Read the model definition and answer for the solid it produces. Units are mm, in the model's axes. A direction names the side the tool comes from. Coordinates: 2 decimals unless noted, no trailing zeros. Write each loop counter-clockwise with the first axis right and the second up, starting at its lowest first coordinate (ties: lowest second). Pieces come first, ordered by that corner, then holes. Notation, with made-up numbers: (19, 29) - (35, 29) arc R18 cw to (35, 34) - close; hole circle Ø2 at (56, 5.5). An arc over 180 degrees is marked (long way). Return JSON: item names as keys, results as strings.
```python
from build123d import *

# Parameters (mm, degrees)
SKETCH_1_W          = 151
SKETCH_1_H          = 95
EXTRUDE_1_DEPTH     = 1.6
SKETCH_2_W          = 41
SKETCH_2_H          = 4.6
EXTRUDE_2_DEPTH     = 151
SKETCH_3_R          = 1.5
CUT_EXTRUDE_1_DEPTH = 179.506134348


with BuildPart() as part:
    # 草图1 → 凸台-拉伸1 (new body)
    with BuildSketch(Plane(origin=(0, 0, 0), x_dir=(1, 0, 0), z_dir=(0, 1, 0))):
        with Locations((75.5, -47.5)):
            Rectangle(SKETCH_1_W, SKETCH_1_H)
    extrude(amount=EXTRUDE_1_DEPTH)

    # 草图2 → 凸台-拉伸2 (add)
    with BuildSketch(Plane.ZY):
        with Locations((47.5, -2.3)):
            Rectangle(SKETCH_2_W, SKETCH_2_H)
    extrude(amount=-EXTRUDE_2_DEPTH)

    # 草图3 → 切除-拉伸1 (cut, through all)
    with BuildSketch(Plane(origin=(0, 1.6, 0), x_dir=(1, 0, 0), z_dir=(0, 1, 0))):
        with Locations(Location((5.5, -5, 0), (0, 0, 270))):
            Circle(SKETCH_3_R)
        with Locations(Location((5.5, -90, 0), (0, 0, 270))):
            Circle(SKETCH_3_R)
        with Locations(Location((145.5, -90, 0), (0, 0, 270))):
            Circle(SKETCH_3_R)
        with Locations(Location((145.5, -5, 0), (0, 0, 270))):
            Circle(SKETCH_3_R)
    extrude(amount=-CUT_EXTRUDE_1_DEPTH, mode=Mode.SUBTRACT)


solid = part.part
```
(1) A cutting plane is placed at D-D (y = -1.5). Determine the outline of the cut face in (x, z).
Answer:
{"outline": "(0, 27) - (151, 27) - (151, 68) - (0, 68) - close"}
(2) Flat-ended cylindrical pins translate along their axes: P1, Ø1.4, axis at x = 44.5, y = -3.5, coming from the +Z side; P2, Ø2.5, axis at x = 5.5, z = 5, coming from the -Y side; P3, Ø1, axis at x = 98, y = -3, coming from the -Z side; P4, Ø4, axis at x = 145.5, z = 90, coming from the -Y side. Find the tip coordinate at first contact, or state that the pin passes through.
Answer:
{"P1": "z = 68", "P2": "through", "P3": "z = 27", "P4": "y = 0"}
(3) Straight lines are drawn through the part: line 1 (Z direction, x = 145.5, y = 0.95); line 2 (X direction, y = 1.05, z = 5); line 3 (Z direction, x = 25, y = -3.75). For each, find the intervals that lie inside material, in ascending order. Write a range as from..to.
Answer:
{"line 1": "0..3.5, 6.5..88.5, 91.5..95", "line 2": "0..4, 7..144, 147..151", "line 3": "27..68"}
(4) A cutting plane is placed at C-C (z = 16). Determine the outline of the cut face in (x, y), and give its area (3 significant figures).
Answer:
{"outline": "(0, 0) - (151, 0) - (151, 1.6) - (0, 1.6) - close", "area": "242 mm²"}
(5) A cutting plane is placed at B-B (z = 90). Determine the outline of the cut face in (x, y).
Answer:
{"outline": "(0, 0) - (4, 0) - (4, 1.6) - (0, 1.6) - close; (7, 0) - (144, 0) - (144, 1.6) - (7, 1.6) - close; (147, 0) - (151, 0) - (151, 1.6) - (147, 1.6) - close"}
(6) Determine the mould class of faces 1 (the face through (151, -1, 48)), 2 (the face through (146.765, 0.811, 90.806)), 3 (the face through (74, 0, 13)) for opening direction X: +X half, -X half, draft (parallel to the pull), parting line (faces both ways), or undercut.
Answer:
{"face 1": "+X half", "face 2": "undercut", "face 3": "draft"}
(7) Which of the six approach directions +Z, -Z, +X, -X, +Y, -Y give full straight-line access (tool end or side, diameter ignored) to faces 4 (the face through (74, 0, 81)), 5 (the face through (74, 1.6, 47)), 6 (the face through (74, -2, 27))?
Answer:
{"face 4": "+Z, +X, -X, -Y", "face 5": "+Z, -Z, +X, -X, +Y", "face 6": "-Z, +X, -X, -Y"}
(8) A cutting plane is placed at A-A (x = 145.5). Determine the outline of the cut face in (y, z).
Answer:
{"outline": "(-4.6, 27) - (0, 27) - (0, 6.5) - (1.6, 6.5) - (1.6, 88.5) - (0, 88.5) - (0, 68) - (-4.6, 68) - close; (0, 0) - (1.6, 0) - (1.6, 3.5) - (0, 3.5) - close; (0, 91.5) - (1.6, 91.5) - (1.6, 95) - (0, 95) - close"}
